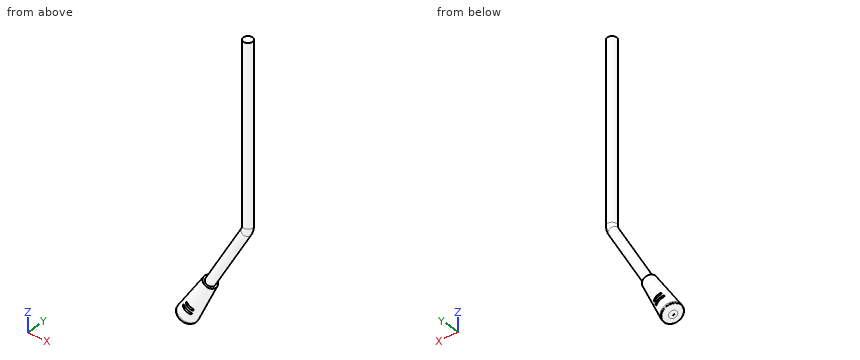
```python
from build123d import *

# Parameters (mm, degrees)
IZIM1_R                           = 3.55
IZIM3_R                           = 5
Y_KSEKLIK_EKSTR_ZYON1_DEPTH       = 35
Y_KSEKLIK_EKSTR_ZYON1_DRAFT       = -4
KES_EKSTR_ZYON1_REACH             = 234.785
KES_EKSTR_ZYON1_DIRECTION_2_REACH = 234.785
IZIM5_R                           = 7.447438418
Y_KSEKLIK_EKSTR_ZYON2_DEPTH       = 2.5
KES_EKSTR_ZYON2_START             = -2.5
KES_EKSTR_ZYON2_DEPTH             = 2.5
SCALE1_SCALE                      = 0.35


# Read off the part's stored shape, not the designer's step: Kes-Ekstrüzyon2
with BuildPart() as part:
    # Süpür1: sweep along a path in Çizim2
    with BuildLine(Plane(origin=(0, 0, 0), x_dir=(1, 0, 0), z_dir=(0, 1, 0))) as s_p_r1_path:
        Line((0, 0), (0, 137.401052942))
        ThreePointArc((0, 137.401052942), (-0.321526794, 139.916436889), (-1.265431279, 142.270068168))
        Line((-1.265431279, 142.270068168), (-29.214091353, 192.407412323))
    # Çizim1 → Süpür1 (sweep)
    with BuildSketch(Plane.XY):
        Circle(IZIM1_R)
    sweep(path=s_p_r1_path.line)


with BuildPart() as y_kseklik_ekstr_zyon1_tool:
    # Çizim3 → Yükseklik-Ekstrüzyon1 (with draft: the straight prism first)
    with BuildSketch(Plane(origin=(-88.754338678, 0, -159.21717935), x_dir=(-0.8734568720516385, 0, 0.48690152255437436), z_dir=(-0.48690152255437436, 0, -0.8734568720516385))):
        with Locations((-68.166213158, 0)):
            Circle(IZIM3_R)
    extrude(amount=Y_KSEKLIK_EKSTR_ZYON1_DEPTH)
    # Yükseklik-Ekstrüzyon1: the draft: its side faces are tilted about the plane it starts from
    y_kseklik_ekstr_zyon1_sides = [y_kseklik_ekstr_zyon1_tool.faces().sort_by_distance(p)[0] for p in [
        (-33.367583638, 0, -210.127415197),
    ]]
    draft(y_kseklik_ekstr_zyon1_sides, Plane(origin=(-88.754338678, 0, -159.21717935), x_dir=(-0.8734568720516385, 0, 0.48690152255437436), z_dir=(-0.48690152255437436, 0, -0.8734568720516385)), Y_KSEKLIK_EKSTR_ZYON1_DRAFT)


with BuildPart() as part_1:
    add(part.part)

    # Yükseklik-Ekstrüzyon1: add y_kseklik_ekstr_zyon1_tool
    add(y_kseklik_ekstr_zyon1_tool.part)

    # Kes-Ekstrüzyon1: up to this cone (the profile starts inside it)
    kes_ekstr_zyon1_end = Plane(origin=(-41.287705224, 0, -214.066373154), z_dir=(-0.48690152255437436, 0, -0.8734568720516385)).offset(-96.300159439) * Cone(1e-06, 23.785643459, 340.150547806, align=(Align.CENTER, Align.CENTER, Align.MIN), mode=Mode.PRIVATE)
    # Çizim4 → Kes-Ekstrüzyon1 (cut, up to the surface)
    with BuildSketch(Plane(origin=(0, 0, 0), x_dir=(1, 0, 0), z_dir=(0, 1, 0)), mode=Mode.PRIVATE) as kes_ekstr_zyon1_sk1:
        with BuildLine():
            Line((-45.209229303, 214.939819091), (-39.968488071, 217.861228226))
            ThreePointArc((-39.968488071, 217.861228226), (-38.824578975, 217.536178458), (-39.149628743, 216.392269362))
            Line((-39.149628743, 216.392269362), (-44.390369975, 213.470860227))
            ThreePointArc((-44.390369975, 213.470860227), (-45.534279071, 213.795909995), (-45.209229303, 214.939819091))
        make_face()
    kes_ekstr_zyon1_tool1 = extrude(kes_ekstr_zyon1_sk1.sketch, amount=-KES_EKSTR_ZYON1_REACH, mode=Mode.PRIVATE) & kes_ekstr_zyon1_end
    add(kes_ekstr_zyon1_tool1.solids().sort_by_distance((-42.179429, 0, -215.666044))[0], mode=Mode.SUBTRACT)
    # Çizim4 → Kes-Ekstrüzyon1 (cut, up to the surface)
    with BuildSketch(Plane(origin=(0, 0, 0), x_dir=(1, 0, 0), z_dir=(0, 1, 0)), mode=Mode.PRIVATE) as kes_ekstr_zyon1_sk2:
        with BuildLine():
            Line((-42.979838494, 211.967397244), (-38.612554134, 214.401904857))
            ThreePointArc((-38.612554134, 214.401904857), (-37.494390623, 214.084170877), (-37.812124603, 212.966007366))
            Line((-37.812124603, 212.966007366), (-42.179408963, 210.531499753))
            ThreePointArc((-42.179408963, 210.531499753), (-43.297572474, 210.849233733), (-42.979838494, 211.967397244))
        make_face()
    kes_ekstr_zyon1_tool2 = extrude(kes_ekstr_zyon1_sk2.sketch, amount=-KES_EKSTR_ZYON1_REACH, mode=Mode.PRIVATE) & kes_ekstr_zyon1_end
    add(kes_ekstr_zyon1_tool2.solids().sort_by_distance((-40.395982, 0, -212.466702))[0], mode=Mode.SUBTRACT)

    # Kes-Ekstrüzyon1 direction 2: up to this cone (the profile starts inside it)
    kes_ekstr_zyon1_direction_2_end = Plane(origin=(-41.287705224, 0, -214.066373154), z_dir=(-0.48690152255437436, 0, -0.8734568720516385)).offset(-96.300159439) * Cone(1e-06, 23.785643459, 340.150547806, align=(Align.CENTER, Align.CENTER, Align.MIN), mode=Mode.PRIVATE)
    # Çizim4 → Kes-Ekstrüzyon1 direction 2 (cut, up to the surface)
    with BuildSketch(Plane(origin=(0, 0, 0), x_dir=(1, 0, 0), z_dir=(0, 1, 0)), mode=Mode.PRIVATE) as kes_ekstr_zyon1_direction_2_sk1:
        with BuildLine():
            Line((-45.209229303, 214.939819091), (-39.968488071, 217.861228226))
            ThreePointArc((-39.968488071, 217.861228226), (-38.824578975, 217.536178458), (-39.149628743, 216.392269362))
            Line((-39.149628743, 216.392269362), (-44.390369975, 213.470860227))
            ThreePointArc((-44.390369975, 213.470860227), (-45.534279071, 213.795909995), (-45.209229303, 214.939819091))
        make_face()
    kes_ekstr_zyon1_direction_2_tool1 = extrude(kes_ekstr_zyon1_direction_2_sk1.sketch, amount=KES_EKSTR_ZYON1_DIRECTION_2_REACH, mode=Mode.PRIVATE) & kes_ekstr_zyon1_direction_2_end
    add(kes_ekstr_zyon1_direction_2_tool1.solids().sort_by_distance((-42.179429, 0, -215.666044))[0], mode=Mode.SUBTRACT)
    # Çizim4 → Kes-Ekstrüzyon1 direction 2 (cut, up to the surface)
    with BuildSketch(Plane(origin=(0, 0, 0), x_dir=(1, 0, 0), z_dir=(0, 1, 0)), mode=Mode.PRIVATE) as kes_ekstr_zyon1_direction_2_sk2:
        with BuildLine():
            Line((-42.979838494, 211.967397244), (-38.612554134, 214.401904857))
            ThreePointArc((-38.612554134, 214.401904857), (-37.494390623, 214.084170877), (-37.812124603, 212.966007366))
            Line((-37.812124603, 212.966007366), (-42.179408963, 210.531499753))
            ThreePointArc((-42.179408963, 210.531499753), (-43.297572474, 210.849233733), (-42.979838494, 211.967397244))
        make_face()
    kes_ekstr_zyon1_direction_2_tool2 = extrude(kes_ekstr_zyon1_direction_2_sk2.sketch, amount=KES_EKSTR_ZYON1_DIRECTION_2_REACH, mode=Mode.PRIVATE) & kes_ekstr_zyon1_direction_2_end
    add(kes_ekstr_zyon1_direction_2_tool2.solids().sort_by_distance((-40.395982, 0, -212.466702))[0], mode=Mode.SUBTRACT)

    # Çizim5 → Yükseklik-Ekstrüzyon2 (add)
    with BuildSketch(Plane(origin=(-105.795891967, 0, -189.788169872), x_dir=(-0.8734568720516382, 0, 0.4869015225543744), z_dir=(-0.4869015225543744, 0, -0.8734568720516382))):
        with Locations((-68.166213158, 0)):
            Circle(IZIM5_R)
    extrude(amount=Y_KSEKLIK_EKSTR_ZYON2_DEPTH)

    # Çizim6 → Kes-Döndür1 (revolve, cut)
    with BuildSketch(Plane(origin=(0, 0, 0), x_dir=(1, 0, 0), z_dir=(0, 1, 0)), mode=Mode.PRIVATE) as kes_d_nd_r1_sk:
        with BuildLine():
            Line((-39.750628377, 226.60457195), (-40.325275653, 227.635436692))
            ThreePointArc((-40.325275653, 227.635436692), (-40.577901157, 227.856858074), (-40.91362857, 227.868441612))
            Line((-40.91362857, 227.868441612), (-44.885136864, 226.60457195))
            Line((-44.885136864, 226.60457195), (-47.472898449, 225.162045025))
            Line((-47.472898449, 225.162045025), (-47.961241176, 226.038087286))
            Line((-47.961241176, 226.038087286), (-40.325275653, 230.294694977))
            Line((-40.325275653, 230.294694977), (-38.62051319, 227.236506781))
            Line((-38.62051319, 227.236506781), (-39.750628377, 226.60457195))
        make_face()
    revolve(kes_d_nd_r1_sk.sketch.rotate(Axis((-47.472898449, 0, -225.162045025), (0.4869015225543754, 0, 0.8734568720516378)), 180), axis=Axis((-47.472898449, 0, -225.162045025), (0.4869015225543754, 0, 0.8734568720516378)), mode=Mode.SUBTRACT)

    # Kes-Ekstrüzyon2 outline → Kes-Ekstrüzyon2 (cut)
    with BuildSketch(Plane(origin=(-107.013145773, 0, -191.971812052), x_dir=(-0.8734568720516384, 0, 0.4869015225543744), z_dir=(-0.4869015225543744, 0, -0.8734568720516384)).offset(KES_EKSTR_ZYON2_START)):
        with BuildLine():
            ThreePointArc((-67.837962268, 0.557294858), (-67.519455213, -0.005510565), (-67.847505862, -0.562807129))
            Line((-67.847505862, -0.562807129), (-67.793032927, -0.594257092))
            ThreePointArc((-67.793032927, -0.594257092), (-67.464977128, 0.025942373), (-67.837962268, 0.620206683))
            Line((-67.837962268, 0.620206683), (-67.837962268, 0.557294858))
        make_face()
        with BuildLine():
            ThreePointArc((-67.847707098, -0.562921038), (-68.494364419, -0.557353528), (-68.812972077, 0.00539495))
            Line((-68.812972077, 0.00539495), (-68.867445011, -0.026055013))
            ThreePointArc((-68.867445011, -0.026055013), (-68.494364418, -0.620259403), (-67.793223859, -0.594376951))
            Line((-67.793223859, -0.594376951), (-67.847707098, -0.562921038))
        make_face()
        with BuildLine():
            ThreePointArc((-68.812970107, 0.00562618), (-68.484819841, 0.562864093), (-67.838161534, 0.557412179))
            Line((-67.838161534, 0.557412179), (-67.838161534, 0.620312106))
            ThreePointArc((-67.838161534, 0.620312106), (-68.539297927, 0.594317029), (-68.867453346, -0.025829733))
            Line((-68.867453346, -0.025829733), (-68.812970107, 0.00562618))
        make_face()
    extrude(amount=KES_EKSTR_ZYON2_DEPTH, mode=Mode.SUBTRACT)


with BuildPart() as part_2:
    # Scale1: scaled about (0, 0, 0)
    add(part_1.part.scale(SCALE1_SCALE))


solid = part_2.part
```
Can you work these out from the model? Positions are in its coordinate system, mm. Give positions to 0.01 mm unless a question says otherwise; leave off trailing zeros. Order: outer loops, then holes, each group sorted by start corner. A loop starts at its lowest first (then second) coordinate and runs counter-clockwise, first axis right, second up. Notation, with made-up numbers: M -16.5,71 L -5.5,71 A19 ccw -5.5,90 Z; hole C 37,5.5 d7. An arc over 180 degrees is marked long. Write item = value, one per line. Start each with the question number.
Q1. Suppose I cut it at A-A (z = -12). Write out the boundary of the cut face in (x, y) (1 decimal).
Q2. I need wall thicknesses on probe 1 along Z at (x, y) = (-15.25, -0.35); probe 2 along X at (y, z) = (1.6, -74); probe 3 along Z at (x, y) = (-14.75, 1.05). Which ranges of each line are inside material? Lowest first, please. Write a range as [from, to].
Q3. Will these pins go through, and if not, where does the flat tip stop? pin 1 Ø2 at (x, y) = (-14, -1.5) entering from +Z; pin 2 Ø1 at (y, z) = (-1, -49.5) entering from -X; pin 3 Ø2 at (x, y) = (-7.5, -1) entering from +Z.
Check result:
q1.outline = C 0,0 d2.5
q2.probe_1 = [-79.45, -75.55], [-74.87, -71.9]
q2.probe_2 = [-15.91, -15.18], [-14.2, -12.17]
q2.probe_3 = [-79.56, -75.83], [-75.15, -74.35], [-73.69, -71.58]
q3.pin_1 = -69.1
q3.pin_2 = -1.69
q3.pin_3 = -58.56
